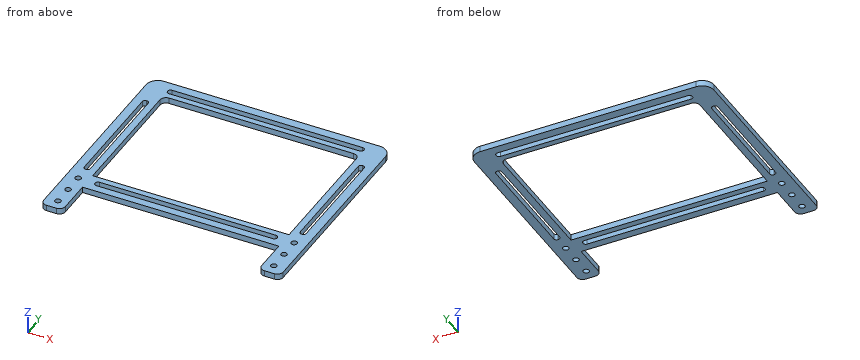
from build123d import *

# Parameters (mm, degrees)
SKETCH1_R           = 1.5
BOSS_EXTRUDE1_DEPTH = 3


with BuildPart() as part:
    # Sketch1 → Boss-Extrude1 (new body)
    with BuildSketch(Plane.XY):
        with BuildLine():
            Line((-61, -52), (-61, 49))
            ThreePointArc((-61, 49), (-59.242640687, 53.242640687), (-55, 55))
            Line((-55, 55), (55, 55))
            ThreePointArc((55, 55), (59.242640687, 53.242640687), (61, 49))
            Line((61, 49), (61, -52))
            ThreePointArc((61, -52), (60.121320344, -54.121320344), (58, -55))
            Line((58, -55), (53, -55))
            ThreePointArc((53, -55), (50.878679656, -54.121320344), (50, -52))
            Line((50, -52), (50, -35))
            Line((50, -35), (-50, -35))
            Line((-50, -35), (-50, -52))
            ThreePointArc((-50, -52), (-50.878679656, -54.121320344), (-53, -55))
            Line((-53, -55), (-58, -55))
            ThreePointArc((-58, -55), (-60.121320344, -54.121320344), (-61, -52))
        make_face()
        with Locations((-55, -49.590163934)):
            Circle(SKETCH1_R, mode=Mode.SUBTRACT)
        with Locations((55, -49.590163934)):
            Circle(SKETCH1_R, mode=Mode.SUBTRACT)
        with Locations((-55, -39.590163934)):
            Circle(SKETCH1_R, mode=Mode.SUBTRACT)
        with Locations((-55, -29.590163934)):
            Circle(SKETCH1_R, mode=Mode.SUBTRACT)
        with Locations((55, -39.590163934)):
            Circle(SKETCH1_R, mode=Mode.SUBTRACT)
        with Locations((55, -29.590163934)):
            Circle(SKETCH1_R, mode=Mode.SUBTRACT)
        with BuildLine():
            Line((-47, 44.5), (47, 44.5))
            ThreePointArc((47, 44.5), (49.121320344, 43.621320344), (50, 41.5))
            Line((50, 41.5), (50, -25))
            Line((50, -25), (-50, -25))
            Line((-50, -25), (-50, 41.5))
            ThreePointArc((-50, 41.5), (-49.121320344, 43.621320344), (-47, 44.5))
        make_face(mode=Mode.SUBTRACT)
        with BuildLine():
            Line((48.6, 50.5), (-48.6, 50.5))
            ThreePointArc((-48.6, 50.5), (-49.589949494, 50.089949494), (-50, 49.1))
            Line((-50, 49.1), (-50, 48.9))
            ThreePointArc((-50, 48.9), (-49.589949494, 47.910050506), (-48.6, 47.5))
            Line((-48.6, 47.5), (48.6, 47.5))
            ThreePointArc((48.6, 47.5), (49.589949494, 47.910050506), (50, 48.9))
            Line((50, 48.9), (50, 49.1))
            ThreePointArc((50, 49.1), (49.589949494, 50.089949494), (48.6, 50.5))
        make_face(mode=Mode.SUBTRACT)
        with BuildLine():
            Line((-55.1, 38.001292496), (-54.9, 38.001292496))
            ThreePointArc((-54.9, 38.001292496), (-53.910050506, 37.59124199), (-53.5, 36.601292496))
            Line((-53.5, 36.601292496), (-53.5, -20.598707504))
            ThreePointArc((-53.5, -20.598707504), (-53.910050506, -21.588656998), (-54.9, -21.998707504))
            Line((-54.9, -21.998707504), (-55.1, -21.998707504))
            ThreePointArc((-55.1, -21.998707504), (-56.089949494, -21.588656998), (-56.5, -20.598707504))
            Line((-56.5, -20.598707504), (-56.5, 36.601292496))
            ThreePointArc((-56.5, 36.601292496), (-56.089949494, 37.59124199), (-55.1, 38.001292496))
        make_face(mode=Mode.SUBTRACT)
        with BuildLine():
            Line((55.1, 38.001292496), (54.9, 38.001292496))
            ThreePointArc((54.9, 38.001292496), (53.910050506, 37.59124199), (53.5, 36.601292496))
            Line((53.5, 36.601292496), (53.5, -20.598707504))
            ThreePointArc((53.5, -20.598707504), (53.910050506, -21.588656998), (54.9, -21.998707504))
            Line((54.9, -21.998707504), (55.1, -21.998707504))
            ThreePointArc((55.1, -21.998707504), (56.089949494, -21.588656998), (56.5, -20.598707504))
            Line((56.5, -20.598707504), (56.5, 36.601292496))
            ThreePointArc((56.5, 36.601292496), (56.089949494, 37.59124199), (55.1, 38.001292496))
        make_face(mode=Mode.SUBTRACT)
        with BuildLine():
            Line((45, -28.090163934), (-45, -28.090163934))
            ThreePointArc((-45, -28.090163934), (-45.989949494, -28.500214441), (-46.4, -29.490163934))
            Line((-46.4, -29.490163934), (-46.4, -29.690163934))
            ThreePointArc((-46.4, -29.690163934), (-45.989949494, -30.680113428), (-45, -31.090163934))
            Line((-45, -31.090163934), (45, -31.090163934))
            ThreePointArc((45, -31.090163934), (45.989949494, -30.680113428), (46.4, -29.690163934))
            Line((46.4, -29.690163934), (46.4, -29.490163934))
            ThreePointArc((46.4, -29.490163934), (45.989949494, -28.500214441), (45, -28.090163934))
        make_face(mode=Mode.SUBTRACT)
    extrude(amount=BOSS_EXTRUDE1_DEPTH)


solid = part.part
Geometry check sheet. Reference: the model listing, model coordinates, mm. Round coordinates to 2 decimals unless told otherwise and drop trailing zeros. Write each loop counter-clockwise with the first axis right and the second up, starting at its lowest first coordinate (ties: lowest second). Pieces come first, ordered by that corner, then holes. Notation, with made-up numbers: (-17.5, -7.5) -> (5.5, -7.5) arc R7 ccw to (5.5, -3.5) -> close; hole circle Ø7 at (-1, 7.5). An arc over 180 degrees is marked (long way). One line per item, written item: value. Start each with the question number.
(1) Cross-section at C-C, the plane y = -45.5. Record the cut outline in (x, z).
(2) Cross-section at D-D, the plane z = 1.1. Give the number of separate pieces and of enclosed holes in the cut face, and give its area (3 significant figures).
(3) Scan lines: line 1 (Y direction, x = 23, z = 2.4); line 2 (X direction, y = 4, z = 1.15); line 3 (Y direction, x = 55, z = 2.85). Record each from-to range of solid material in increasing order. Write a range as [from, to].
(4) Cross-section at B-B, the plane y = -1. Record the cut outline in (x, z), and give its area (3 significant figures).
(5) Cross-section at A-A, the plane x = -24.5. Record the cut outline in (y, z).
(6) Go/stop test with flat-tipped pins: pin 1 Ø0.9 at (x, z) = (22.5, 2) entering from -Y; pin 2 Ø1.8 at (x, y) = (55, -49.59) entering from +Z. Record where each tip stops, or that it passes through.
Answer:
1. outline: (-61, 0) -> (-50, 0) -> (-50, 3) -> (-61, 3) -> close; (50, 0) -> (61, 0) -> (61, 3) -> (50, 3) -> close
2. separate pieces: 1
2. enclosed holes: 11
2. area: 3,480 mm²
3. line 1: [-35, -31.09], [-28.09, -25], [44.5, 47.5], [50.5, 55]
3. line 2: [-61, -56.5], [-53.5, -50], [50, 53.5], [56.5, 61]
3. line 3: [-55, -51.09], [-48.09, -41.09], [-38.09, -31.09], [-28.09, -22], [38, 55]
4. outline: (-61, 0) -> (-56.5, 0) -> (-56.5, 3) -> (-61, 3) -> close; (-53.5, 0) -> (-50, 0) -> (-50, 3) -> (-53.5, 3) -> close; (50, 0) -> (53.5, 0) -> (53.5, 3) -> (50, 3) -> close; (56.5, 0) -> (61, 0) -> (61, 3) -> (56.5, 3) -> close
4. area: 48.0 mm²
5. outline: (-35, 0) -> (-31.09, 0) -> (-31.09, 3) -> (-35, 3) -> close; (-28.09, 0) -> (-25, 0) -> (-25, 3) -> (-28.09, 3) -> close; (44.5, 0) -> (47.5, 0) -> (47.5, 3) -> (44.5, 3) -> close; (50.5, 0) -> (55, 0) -> (55, 3) -> (50.5, 3) -> close
6. pin 1: y = -35
6. pin 2: through
